Check sheet for the modelled part. Datum: model origin and axes. Units: mm. Face numbers are marked on the shaded views. A direction names the side the tool comes from. Coordinates: 2 decimals unless noted, no trailing zeros. Write each loop counter-clockwise with the first axis right and the second up, starting at its lowest first coordinate (ties: lowest second). Pieces come first, ordered by that corner, then holes. Notation, with made-up numbers: M 40,81 L 60,81 A9 cw 60,98 Z; hole C 84,14.25 d4. An arc over 180 degrees is marked long. Answer as CSV lines item,"result". Start each with the question number.
Q1. Depth check by flat-ended pin: pin 1 Ø1.3 at (x, z) = (-3.5, 1) entering from +Y; pin 2 Ø3 at (y, z) = (-6.5, -2) entering from -X; pin 3 Ø2 at (y, z) = (-7, 1) entering from +X; pin 4 Ø1 at (y, z) = (-6.5, -2.5) entering from +X. Enter the tip coordinate at first touch or a pass-through.
Q2. Sectioned sample at A-A, the plane y = -8.75. Record the cut outline in (x, z).
Q3. Sectioned sample at C-C, the plane z = 3.75. Record the cut outline in (x, y).
Q4. Sectioned sample at D-D, the plane y = -2.75. Record the cut outline in (x, z).
Q5. Thickness scan on line 1 along X through (y, z) = (-9.5, -1.75); line 2 along X through (y, z) = (-3.5, 3.25); line 3 along Z through (x, y) = (-1, -5.25). Record the ranges inside material, lowest first. Write a range as from..to.
Q6. Mould release check, pull along X, two halves, no side actions. Record for the marked faces 1, 2 and 3: pulls with the +X half, pulls with the -X half, needs draft (parallel to the pull), parting line crosses it, or undercut.
Q7. Access from +Z, -Z, +X, -X, +Y, -Y to the whole of each face (thin tool, end or side, straight path). Record for the marked faces 4, 5, 6, 7 and 8.
Q8. Sectioned sample at B-B, the plane y = -1.5. Record the cut outline in (x, z), then the cut area to 3 significant figures.
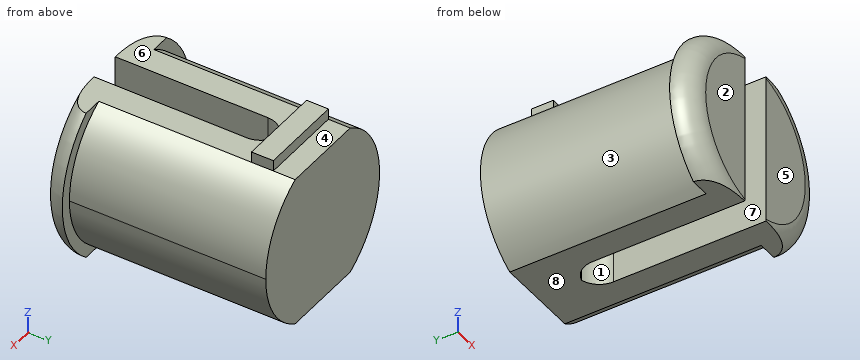
from build123d import *

# Parameters (mm, degrees)
F1_DEPTH    = 10
F3_DEPTH    = 1
F2_W        = 1.5
F2_H        = 7
F4_DEPTH    = 8
F6_T1_DEPTH = 7
F6_T4_ANGLE = 165.8100193305
F6_T6_ANGLE = 165.8100193305
F7_DEPTH    = 0.5


# Not quite as in the source:
# - a fillet or chamfer that OpenCascade refuses, or shapes differently, is made with other operations: its cross-section is extruded or revolved along the edge and cut away or added


with BuildPart() as f1:
    # F0 (on Front) → F1 (new body)
    with BuildSketch(Plane.XZ):
        with BuildLine():
            ThreePointArc((1.9364916731, -3.5), (3.4457195687, -2.0315060063), (4, 0))
            ThreePointArc((4, 0), (3.4457195687, 2.0315060063), (1.9364916731, 3.5))
            Line((1.9364916731, 3.5), (-1.9364916731, 3.5))
            ThreePointArc((-1.9364916731, 3.5), (-4, 0), (-1.9364916731, -3.5))
            Line((-1.9364916731, -3.5), (1.9364916731, -3.5))
        make_face()
    extrude(amount=F1_DEPTH)

    # F2 (on face) → F3 (join)
    with BuildSketch(Plane.XZ.offset(10)):
        with BuildLine():
            Line((-1.9364916731, 3.5), (-2.8284271247, 3.5))
            ThreePointArc((-2.8284271247, 3.5), (-4.5, 0), (-2.8284271247, -3.5))
            Line((-2.8284271247, -3.5), (-1.9364916731, -3.5))
            ThreePointArc((-1.9364916731, -3.5), (-4, 0), (-1.9364916731, 3.5))
        make_face()
        with BuildLine():
            ThreePointArc((2.8284271247, -3.5), (4.0606601718, -1.9393398282), (4.5, 0))
            ThreePointArc((4.5, 0), (4.0606601718, 1.9393398282), (2.8284271247, 3.5))
            Line((2.8284271247, 3.5), (1.9364916731, 3.5))
            ThreePointArc((1.9364916731, 3.5), (4, 0), (1.9364916731, -3.5))
            Line((1.9364916731, -3.5), (2.8284271247, -3.5))
        make_face()
    extrude(amount=-F3_DEPTH)

    # F2 (on face) → F4 (cut)
    with BuildSketch(Plane.XZ.offset(10)):
        Rectangle(F2_W, F2_H)
    extrude(amount=-F4_DEPTH, mode=Mode.SUBTRACT)

    # F6: fillet of radius 1 on 4 edges, made by hand

    # F6_s2 → F6_t1 (join)
    with BuildSketch(Plane.XY.offset(-3.5)):
        with BuildLine():
            ThreePointArc((0.25, -2), (-0.4571067812, -2.2928932188), (-0.75, -3))
            Line((-0.75, -3), (-0.75, -2))
            Line((-0.75, -2), (0.25, -2))
        make_face()
        with BuildLine():
            ThreePointArc((0.75, -3), (0.4571067812, -2.2928932188), (-0.25, -2))
            Line((-0.25, -2), (0.75, -2))
            Line((0.75, -2), (0.75, -3))
        make_face()
    extrude(amount=F6_T1_DEPTH)

    # F6_s3 → F6_t4 (revolve, cut)
    with BuildSketch(Plane(origin=(0, 0, 0), x_dir=(0, 1, 0), z_dir=(0.9923427412, 0, 0.1235147116))):
        with BuildLine():
            ThreePointArc((-10, 3.5), (-9.7071067812, 4.2071067812), (-9, 4.5))
            Line((-9, 4.5), (-10, 4.5))
            Line((-10, 4.5), (-10, 3.5))
        make_face()
    revolve(axis=Axis((0, -10, 0), (0, -1, 0)), revolution_arc=F6_T4_ANGLE, mode=Mode.SUBTRACT)

    # F6_s5 → F6_t6 (revolve, cut)
    with BuildSketch(Plane(origin=(0, 0, 0), x_dir=(0, 1, 0), z_dir=(-0.9923427412, 0, -0.1235147116))):
        with BuildLine():
            ThreePointArc((-9, 4.5), (-9.7071067812, 4.2071067812), (-10, 3.5))
            Line((-10, 3.5), (-10, 4.5))
            Line((-10, 4.5), (-9, 4.5))
        make_face()
    revolve(axis=Axis((0, -10, 0), (0, -1, 0)), revolution_arc=F6_T6_ANGLE, mode=Mode.SUBTRACT)

    # F5 (on face) → F7 (join)
    with BuildSketch(Plane.XY.offset(3.5)):
        Polygon((-1.9364916731, -1), (-1.9364916731, -2), (-0.75, -2), (0.75, -2), (1.9364916731, -2), (1.9364916731, -1), align=None)
    extrude(amount=F7_DEPTH)


solid = f1.part
Output:
1,pin 1,"stops at y = 0"
1,pin 2,"stops at x = -3.97"
1,pin 3,"stops at x = 4"
1,pin 4,"stops at x = 3.46"
2,outline,"M -1.94,-3.5 L -0.75,-3.5 L -0.75,3.5 L -1.94,3.5 A4 ccw Z; M 0.75,-3.5 L 1.94,-3.5 A4 ccw 1.94,3.5 L 0.75,3.5 Z"
3,outline,"M -1.94,-2 L 1.94,-2 L 1.94,-1 L -1.94,-1 Z"
4,outline,"M -1.94,-3.5 L -0.72,-3.5 L -0.72,3.5 L -1.94,3.5 A4 ccw Z; M 0.72,-3.5 L 1.94,-3.5 A4 ccw 1.94,3.5 L 0.72,3.5 Z"
5,line 1,"x = -4..-0.75, 0.75..4"
5,line 2,"x = -2.33..-0.75, 0.75..2.33"
5,line 3,"z = -3.5..3.5"
6,face 1,"undercut"
6,face 2,"needs draft"
6,face 3,"pulls with the -X half"
7,face 4,"+Z, +X, -X, +Y"
7,face 5,"+Z, -Z, +X, -X, -Y"
7,face 6,"+Z, +X, -X, -Y"
7,face 7,"+Z, -Z, -Y"
7,face 8,"-Z, +X, -X, +Y, -Y"
8,outline,"M -1.94,-3.5 L 1.94,-3.5 A4 ccw 1.94,3.5 L 1.94,4 L -1.94,4 L -1.94,3.5 A4 ccw Z"
8,area,"49.6 mm^2"
